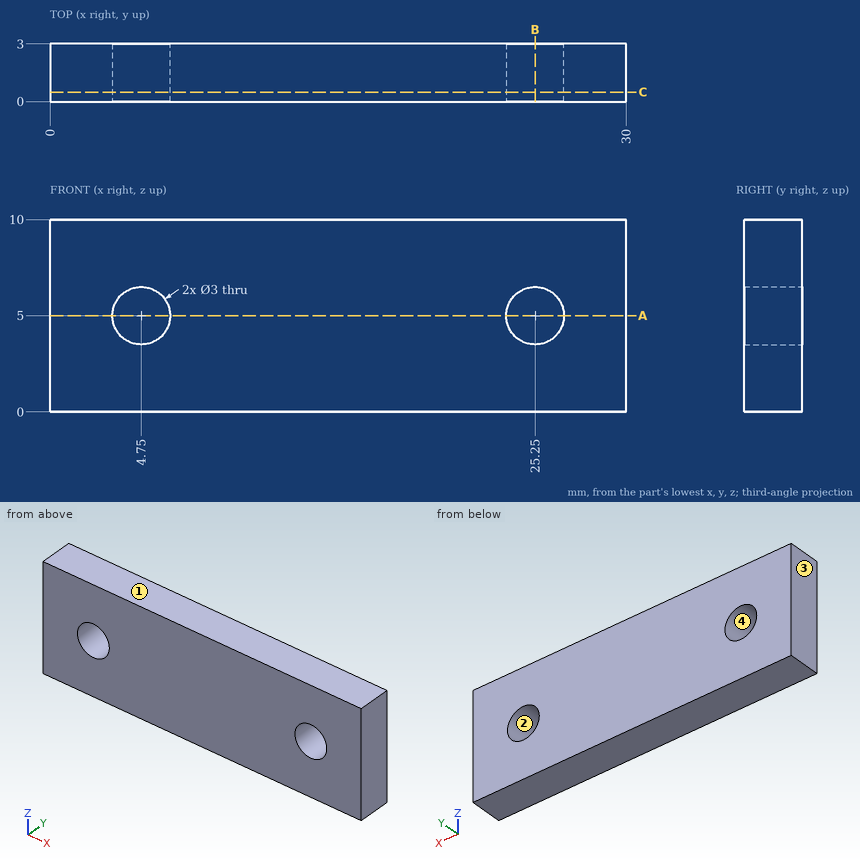
Job drawing, mm, ordinate dimensions from the low corner. One solid piece. Coordinates: 2 decimals unless noted, no trailing zeros. Write each loop counter-clockwise with the first axis right and the second up, starting at its lowest first coordinate (ties: lowest second). Pieces come first, ordered by that corner, then holes. Notation, with made-up numbers: (6, 49.25) -> (33, 49.25) arc R12 ccw to (33, 55.25) -> close; hole circle Ø4 at (21.5, 11). An arc over 180 degrees is marked (long way). Use CSV: the item, a comma, the result in double quotes. Start each with the question number.
Item 1: Two-plate mould, pull along X, no slides. Class the marked faces 1, 2, 3 and 4: +X half, -X half, draft (parallel to the pull), parting line (faces both ways), or undercut.
Item 2: Band-saw the part on C-C, the plane y = 0.5. Write the cut outline in (x, z), plus the area to 3 significant figures.
Item 3: Band-saw the part on B-B, the plane x = 25.25. Write the cut outline in (y, z), plus the area to 3 significant figures.
Item 4: Band-saw the part on A-A, the plane z = 5. Write the cut outline in (x, y).
Item 5: Wall check: probe 1 along Z at (x, y) = (25.25, 1.75); probe 2 along Z at (x, y) = (4.25, 1.45). Give the ranges that are in metal, low to high.
Response values:
1,face 1,"draft"
1,face 2,"undercut"
1,face 3,"-X half"
1,face 4,"undercut"
2,outline,"(0, 0) -> (30, 0) -> (30, 10) -> (0, 10) -> close; hole circle Ø3 at (4.75, 5); hole circle Ø3 at (25.25, 5)"
2,area,"286 mm2"
3,outline,"(0, 0) -> (3, 0) -> (3, 3.5) -> (0, 3.5) -> close; (0, 6.5) -> (3, 6.5) -> (3, 10) -> (0, 10) -> close"
3,area,"21.0 mm2"
4,outline,"(0, 0) -> (3.25, 0) -> (3.25, 3) -> (0, 3) -> close; (6.25, 0) -> (23.75, 0) -> (23.75, 3) -> (6.25, 3) -> close; (26.75, 0) -> (30, 0) -> (30, 3) -> (26.75, 3) -> close"
5,probe 1,"z = 0 to 3.5, 6.5 to 10"
5,probe 2,"z = 0 to 3.59, 6.41 to 10"
